For this review, take the finished solid that the model builds, in its own axes (mm). A direction names the side the tool comes from. Round coordinates to 2 decimals unless told otherwise and drop trailing zeros. Write each loop counter-clockwise with the first axis right and the second up, starting at its lowest first coordinate (ties: lowest second). Pieces come first, ordered by that corner, then holes. Notation, with made-up numbers: (23, 83.5) -> (65, 83.5) arc R21 cw to (65, 122.5) -> close; hole circle Ø6 at (78, 79). An arc over 180 degrees is marked (long way). Write item = value, one per line. Start each with the question number.
```python
from build123d import *

# Parameters (mm, degrees)
F0_W     = 17.5
F0_H     = 120
F0_W_2   = 5
F1_DEPTH = 5
F2_W     = 5
F2_H     = 100
F3_DEPTH = 5
F4_D     = 4.5
F4_DEPTH = 17
F4_TIP   = 1.3519363928


with BuildPart() as f1:
    # F0 (on Front) → F1 (new body)
    with BuildSketch(Plane.XZ):
        with Locations((-11.25, 0)):
            Rectangle(F0_W, F0_H)
        with BuildLine():
            Line((-7.75, -35), (-7.75, -55))
            ThreePointArc((-7.75, -55), (-10, -57.25), (-12.25, -55))
            Line((-12.25, -55), (-12.25, -35))
            ThreePointArc((-12.25, -35), (-10, -32.75), (-7.75, -35))
        make_face(mode=Mode.SUBTRACT)
        Rectangle(F0_W_2, F0_H)
        with Locations((11.25, 0)):
            Rectangle(F0_W, F0_H)
        with BuildLine():
            Line((12.25, -35), (12.25, -55))
            ThreePointArc((12.25, -55), (10, -57.25), (7.75, -55))
            Line((7.75, -55), (7.75, -35))
            ThreePointArc((7.75, -35), (10, -32.75), (12.25, -35))
        make_face(mode=Mode.SUBTRACT)
    extrude(amount=F1_DEPTH)

    # F2 (on face) → F3 (join)
    with BuildSketch(Plane.XZ.offset(5)):
        Rectangle(F2_W, F2_H)
    extrude(amount=F3_DEPTH)

    # F4
    with Locations(Plane(origin=(0, 0, 0), x_dir=(1, 0, 0), z_dir=(0, 1, 0))):
        with Locations((10, -50), (-10, -50)):
            Hole(F4_D / 2, depth=F4_DEPTH)
            with Locations((0, 0, -(F4_DEPTH + F4_TIP / 2))):  # 118° drill point
                Cone(0, F4_D / 2, F4_TIP, mode=Mode.SUBTRACT)


solid = f1.part
```
1. Clearance check with flat-ended pins moving along their axes: pin 1 Ø1.5 at (y, z) = (-7, -6.5) entering from +X; pin 2 Ø5.5 at (x, y) = (-1, -8.5) entering from +Z; pin 3 Ø3 at (x, z) = (14, 43) entering from -Y; pin 4 Ø3.5 at (x, z) = (10, 50) entering from +Y. State where each tip first meets the part, or that it passes through.
2. Consider section A-A, the plane z = -52.5. Give the boundary of the cut face in (x, y).
3. Wall thickness on L1, parallel to X at y = -3.15, z = 50; L2, parallel to Z at x = -10, y = -3.8; L3, parallel to X at y = -3.25, z = -34: over which ranges is each line inside the solid? List them lowest first. Write a range as from..to.
4. Consider section C-C, the plane y = -2.5. Give the boundary of the cut face in (x, z).
5. Draft analysis for pull direction X (two halves, no side actions). For faces 5 (the flat face through (7.75, -2, -45)), 6 (the flat face through (-20, -2, -1)), 7 (the flat face through (2.5, -7, -1)), 8 (the flat face through (0, -7, -50)), state which applies: +X half, -X half, draft (parallel to the pull), parting line (faces both ways), or undercut.
6. Consider section D-D, the plane x = 1. Give the boundary of the cut face in (y, z).
7. Consider section B-B, the plane x = -10. Give the boundary of the cut face in (y, z), then the cut area to 3 significant figures.
8. Machinability: for faces 1 (the flat face through (20, -2, -1)), 2 (the flat face through (-2.5, -7, -1)), 3 (the flat face through (0, -7, 50)), 4 (the flat face through (12.25, -2, -45)), which of the approach directions +Z, -Z, +X, -X, +Y, -Y give a long, thin tool a straight path to every point of the face, cutting with its end or side? Answer none if there is none.
Outcome:
q1.pin_1 = 2.5
q1.pin_2 = 50
q1.pin_3 = -5
q1.pin_4 = through
q2.outline = (-20, -5) -> (-12.25, -5) -> (-12.25, 0) -> (-20, 0) -> close; (-7.75, -5) -> (7.75, -5) -> (7.75, 0) -> (-7.75, 0) -> close; (12.25, -5) -> (20, -5) -> (20, 0) -> (12.25, 0) -> close
q3.L1 = -20..-12.25, -7.75..7.75, 12.25..20
q3.L2 = -60..-57.25, -32.75..47.75, 52.25..60
q3.L3 = -20..-12.02, -7.98..7.98, 12.02..20
q4.outline = (-20, -60) -> (20, -60) -> (20, 60) -> (-20, 60) -> close; hole (-12.25, -55) arc R2.25 ccw to (-7.75, -55) -> (-7.75, -35) arc R2.25 ccw to (-12.25, -35) -> close; hole circle Ø4.5 at (-10, 50); hole (7.75, -55) arc R2.25 ccw to (12.25, -55) -> (12.25, -35) arc R2.25 ccw to (7.75, -35) -> close; hole circle Ø4.5 at (10, 50)
q5.face_5 = undercut
q5.face_6 = -X half
q5.face_7 = +X half
q5.face_8 = draft
q6.outline = (-10, -50) -> (-5, -50) -> (-5, -60) -> (0, -60) -> (0, 60) -> (-5, 60) -> (-5, 50) -> (-10, 50) -> close
q7.outline = (-5, -60) -> (0, -60) -> (0, -57.25) -> (-5, -57.25) -> close; (-5, -32.75) -> (0, -32.75) -> (0, 47.75) -> (-5, 47.75) -> close; (-5, 52.25) -> (0, 52.25) -> (0, 60) -> (-5, 60) -> close
q7.area = 455 mm2
q8.face_1 = +Z, -Z, +X, +Y, -Y
q8.face_2 = +Z, -Z, -X, -Y
q8.face_3 = +Z, +X, -X, -Y
q8.face_4 = +Y, -Y
